Can you work these out from the drawing? Everything is in mm from the part's minimum corner. A direction names the side the tool comes from. Round coordinates to 2 decimals unless told otherwise and drop trailing zeros. Write each loop counter-clockwise with the first axis right and the second up, starting at its lowest first coordinate (ties: lowest second). Pieces come first, ordered by that corner, then holes. Notation, with made-up numbers: (25.25, 1.25) - (32.25, 1.25) arc R37 ccw to (32.25, 40.25) - close; hole circle Ø8 at (82, 54). An arc over 180 degrees is marked (long way). One line per item, written item: value. Start each with the question number.
(1) I want a section at A-A on x = 14.5. List the corners of the cut face in (y, z) for me.
(2) I want a section at C-C on z = 10.5. List the corners of the cut face in (x, y) for me.
(3) I'm going to push flat-ended pins straight in: pin 1 Ø4.5 at (x, y) = (42.926, 54.991) entering from +Z; pin 2 Ø2 at (y, z) = (14, 2) entering from -X; pin 3 Ø6 at (y, z) = (23.5, 2) entering from +X. Where does each tip first touch, or does it pass through?
(4) I want a section at B-B on y = 16. List the corners of the cut face in (x, z) for me, plus the area to 3 significant figures.
(5) If I drill on L1, parallel to Y at x = 35.5, z = 5.25; L2, parallel to Y at x = 28.5, z = 10.5; L3, parallel to Z at x = 37, y = 40, over which ranges is the centre line in solid material (lowest first)? Write a range as from..to.
(6) I want a section at D-D on z = 1.5. List the corners of the cut face in (x, y) for me (3 decimals).
(7) Thinking about a two-plate mould opening in X: for the marked faces 1 and 2, which applies, +X half, -X half, draft (parallel to the pull), parting line (faces both ways), or undercut?
(8) On a 3-axis mill with a long thin cutter (end or side, diameter ignored), from which of +Z, -Z, +X, -X, +Y, -Y can I reach the whole of each face in a straight line? I mean the marked faces 3, 4 and 5. Say none if no direction works.
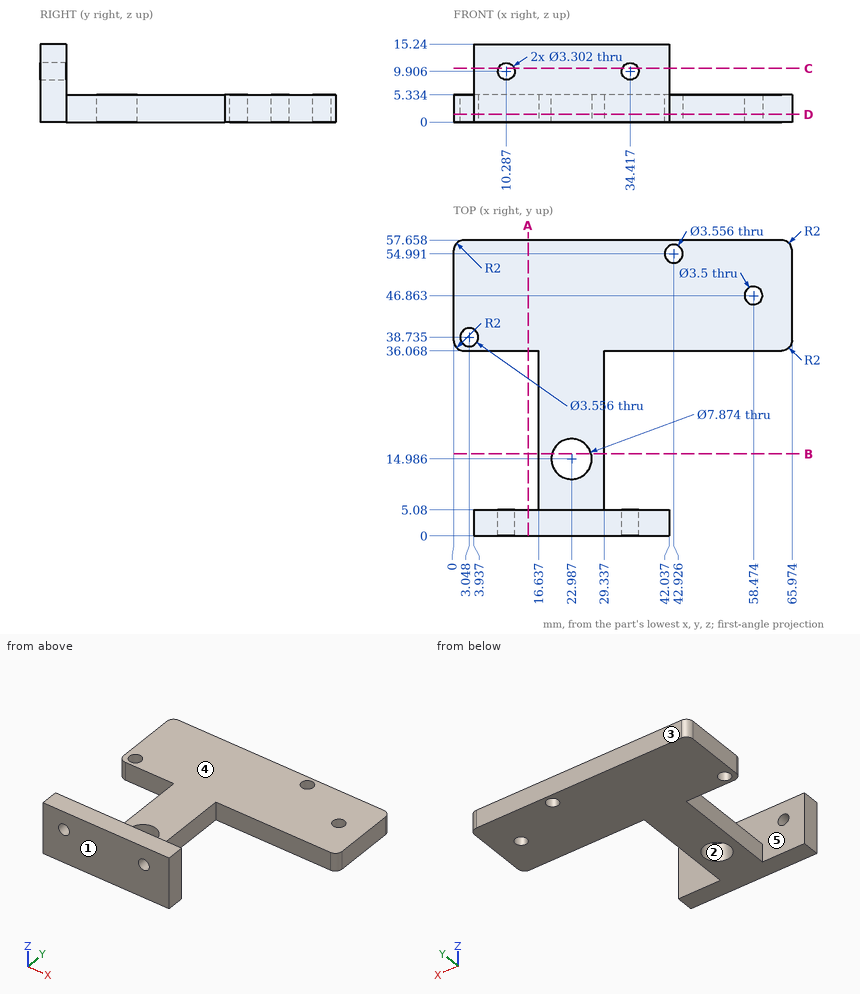
Established:
1. outline: (0, 0) - (5.08, 0) - (5.08, 15.24) - (0, 15.24) - close; (36.07, 0) - (57.66, 0) - (57.66, 5.33) - (36.07, 5.33) - close
2. outline: (3.94, 0) - (8.75, 0) - (8.75, 5.08) - (3.94, 5.08) - close; (11.83, 0) - (32.88, 0) - (32.88, 5.08) - (11.83, 5.08) - close; (35.96, 0) - (42.04, 0) - (42.04, 5.08) - (35.96, 5.08) - close
3. pin 1: z = 5.33
3. pin 2: x = 16.64
3. pin 3: x = 29.34
4. outline: (16.64, 0) - (19.18, 0) - (19.18, 5.33) - (16.64, 5.33) - close; (26.79, 0) - (29.34, 0) - (29.34, 5.33) - (26.79, 5.33) - close
4. area: 27.2 mm2
5. L1: 0..5.08, 36.07..57.66
5. L2: 0..5.08
5. L3: 0..5.33
6. outline: (0, 38.068) arc R2 ccw to (2, 36.068) - (16.637, 36.068) - (16.637, 5.08) - (3.937, 5.08) - (3.937, 0) - (42.037, 0) - (42.037, 5.08) - (29.337, 5.08) - (29.337, 36.068) - (63.974, 36.068) arc R2 ccw to (65.974, 38.068) - (65.974, 55.658) arc R2 ccw to (63.974, 57.658) - (2, 57.658) arc R2 ccw to (0, 55.658) - close; hole circle Ø3.556 at (3.048, 38.735); hole circle Ø7.874 at (22.987, 14.986); hole circle Ø3.556 at (42.926, 54.991); hole circle Ø3.5 at (58.474, 46.863)
7. face 1: draft
7. face 2: undercut
8. face 3: +Z, -Z, +X, -X, +Y
8. face 4: +Z, +X, -X, +Y
8. face 5: +Z
